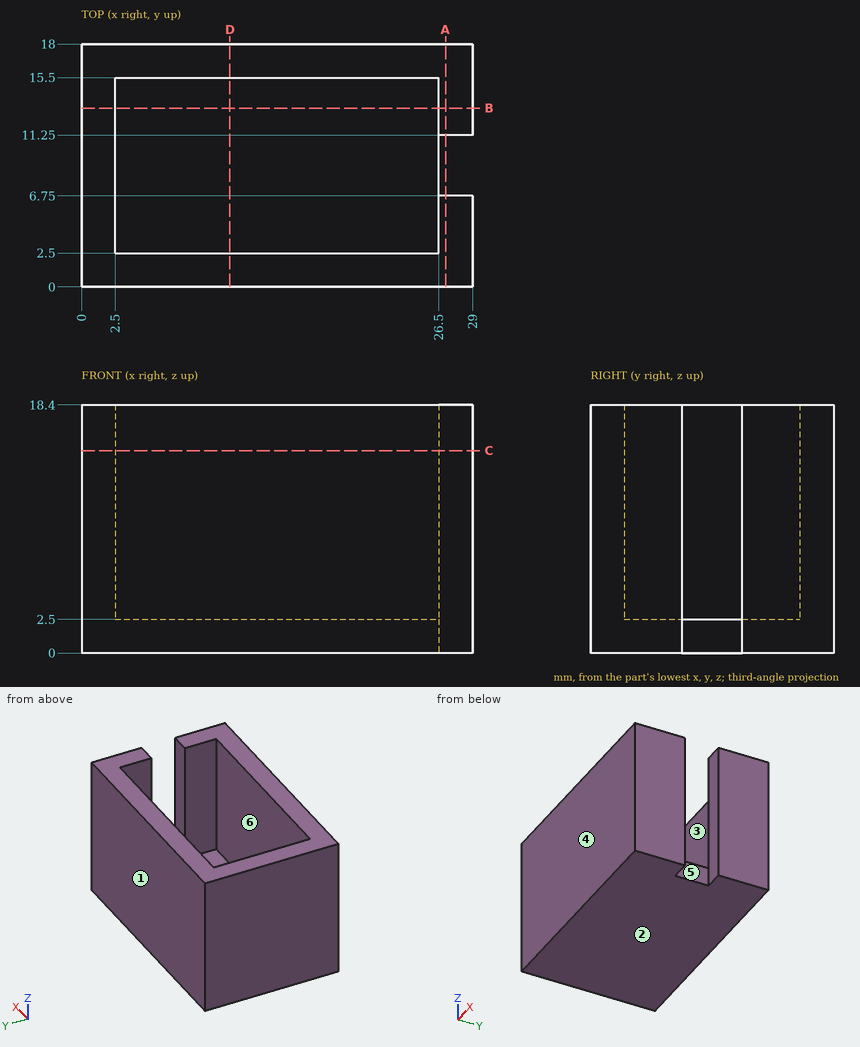
Study the drawing (mm; zero at the part's minimum x, y, z) and answer. A direction names the side the tool comes from. Coordinates: 2 decimals unless noted, no trailing zeros. Loops run counter-clockwise (first coordinate to the right, second up) from the corner with the lowest first, then second, coordinate; pieces in that order, holes last. Notation, with made-up numbers: M 57,39.5 L 68,39.5 A27 cw 68,73.5 Z; hole C 29,88.25 d9. An arc over 180 degrees is marked long. Answer in a Markdown table with one row per item. Add a question column.
1. Find section C-C, the plane z = 15. Write down the section's boundary in (x, y), then the cut area to 3 significant figures.
2. Flat-ended cylindrical pins translate along their axes: P1, Ø1.2, axis at y = 10, z = 1.5, coming from the +X side; P2, Ø5, axis at x = 19.5, y = 5.5, coming from the +Z side; P3, Ø2, axis at y = 9.5, z = 9, coming from the +X side. Find the tip coordinate at first contact, or state that the pin passes through.
3. A tool of negligible diameter and unlimited length cuts with its end or side. For the marked faces 4, 5 and 6, from which of +Z, -Z, +X, -X, +Y, -Y can it reach the whole face along a straight path? Write none if from no direction.
4. The mould has two halves that part along Y. Classify the marked faces 1, 2 and 3: pulls with the +Y half, pulls with the -Y half, needs draft (parallel to the pull), parting line crosses it, or undercut.
5. Find section B-B, the plane y = 13.25. Write down the section's boundary in (x, z), then the cut area to 3 significant figures.
6. Find section D-D, the plane x = 11. Write down the section's boundary in (y, z).
7. Consider L1, parallel to Y at x = 3, z = 15.5; L2, parallel to X at y = 13.5, z = 10.75; L3, parallel to X at y = 10, z = 2. Determine where each line is inside the solid, lowest interval first.
8. Find section A-A, the plane x = 27. Write down the section's boundary in (y, z).
Reported:
| question | item | result |
|---|---|---|
| 1 | outline | M 0,0 L 29,0 L 29,6.75 L 26.5,6.75 L 26.5,2.5 L 2.5,2.5 L 2.5,15.5 L 26.5,15.5 L 26.5,11.25 L 29,11.25 L 29,18 L 0,18 Z |
| 1 | area | 199 mm^2 |
| 2 | P1 | stops at x = 26.5 |
| 2 | P2 | stops at z = 2.5 |
| 2 | P3 | stops at x = 2.5 |
| 3 | face 4 | +Z, -Z, +X, -X, -Y |
| 3 | face 5 | +Z, -Z, +X |
| 3 | face 6 | +Z |
| 4 | face 1 | pulls with the +Y half |
| 4 | face 2 | needs draft |
| 4 | face 3 | undercut |
| 5 | outline | M 0,0 L 29,0 L 29,18.4 L 26.5,18.4 L 26.5,2.5 L 2.5,2.5 L 2.5,18.4 L 0,18.4 Z |
| 5 | area | 152 mm^2 |
| 6 | outline | M 0,0 L 18,0 L 18,18.4 L 15.5,18.4 L 15.5,2.5 L 2.5,2.5 L 2.5,18.4 L 0,18.4 Z |
| 7 | L1 | y = 0 to 2.5, 15.5 to 18 |
| 7 | L2 | x = 0 to 2.5, 26.5 to 29 |
| 7 | L3 | x = 0 to 26.5 |
| 8 | outline | M 0,0 L 6.75,0 L 6.75,18.4 L 0,18.4 Z; M 11.25,0 L 18,0 L 18,18.4 L 11.25,18.4 Z |
